The model under review builds one solid part; all positions refer to its coordinate system, in mm. A direction names the side the tool comes from. Round coordinates to 2 decimals unless told otherwise and drop trailing zeros. Loops run counter-clockwise (first coordinate to the right, second up) from the corner with the lowest first, then second, coordinate; pieces in that order, holes last. Notation, with made-up numbers: M 63.5,66 L 76.5,66 A28 cw 76.5,101 Z; hole C -1.75,0 d8. An arc over 180 degrees is marked long. Return JSON: item names as keys, results as strings. Group by question number.
Q1. For faces 1 (the face through (6, 9, 26.5)), 2 (the face through (6, 16, 22.3)), 3 (the face through (6, 0, 8)), list the 3-axis set-ups (+Z, -Z, +X, -X, +Y, -Y) from which the entire face can be reached by the end or side of a thin tool; tool diameter is ignored.
Q2. Consider section C-C (x = 10.75). State the section outline as (y, z) points.
Q3. Consider section A-A (z = 7). State the section outline as (x, y) points, and give its area (3 significant figures).
Q4. Consider section B-B (x = 5.5). Count the separate pieces of the cut face and the enclosed holes in it, and give its area (3 significant figures).
Q5. Clearance check with flat-ended pins moving along their axes: pin 1 Ø6 at (x, y) = (4, -2) entering from +Z; pin 2 Ø2.5 at (x, y) = (3.5, -2) entering from -Z; pin 3 Ø2.5 at (x, y) = (5, 23.5) entering from +Z; pin 4 Ø1.6 at (x, y) = (6, 25) entering from -Z. State where each tip first meets the part, or that it passes through.
Q6. Consider section D-D (z = 23). State the section outline as (x, y) points, and give its area (3 significant figures).
Q7. To check wall thickness, follow line 1 along Y through (x, z) = (5.9, 17.15); line 2 along X through (y, z) = (-2.6, 16.75); line 3 along Z through (x, y) = (1.25, 7). State the ranges of each line that lie inside material, in increasing order.
from build123d import *

# Parameters (mm, degrees)
F0_W     = 11.8
F0_H     = 22.5
F1_DEPTH = 22.3
F4_DEPTH = 2.5
F6_DEPTH = 4.2
F7_R     = 2.45
F8_DEPTH = 3
F9_R     = 0.5


with BuildPart() as f1:
    # F0 (on Top) → F1 (new body)
    with BuildSketch(Plane.XY):
        with Locations((5.9, 11.25)):
            Rectangle(F0_W, F0_H)
    extrude(amount=F1_DEPTH)

    # F3 (on offset) → F4 (join)
    with BuildSketch(Plane.XY.offset(16)):
        Polygon((11.8, 27.4), (0, 27.4), (0, 11.25), (0, -4.9), (11.8, -4.9), align=None)
        with BuildLine():
            ThreePointArc((6.9, -2.6), (5.1928932188, -3.3071067812), (5.9, -1.6))
            ThreePointArc((5.9, -1.6), (6.6071067812, -1.8928932188), (6.9, -2.6))
        make_face(mode=Mode.SUBTRACT)
        with BuildLine():
            ThreePointArc((6.9, 25.1), (6.6071067812, 24.3928932188), (5.9, 24.1))
            ThreePointArc((5.9, 24.1), (5.1928932188, 25.8071067812), (6.9, 25.1))
        make_face(mode=Mode.SUBTRACT)
    extrude(amount=F4_DEPTH)

    # F5 (on face) → F6 (join)
    with BuildSketch(Plane.XY.offset(22.3)):
        with BuildLine():
            ThreePointArc((3.2367553675, 11.1647058824), (2.8099468719, 0.8739108976), (11.8, 5.9))
            ThreePointArc((11.8, 5.9), (10.9260891024, 8.9900531281), (8.5632446325, 11.1647058824))
            ThreePointArc((8.5632446325, 11.1647058824), (5.9, 9.1), (3.2367553675, 11.1647058824))
        make_face()
        with BuildLine():
            ThreePointArc((3.2367553675, 11.1647058824), (5.9, 9.1), (8.5632446325, 11.1647058824))
            ThreePointArc((8.5632446325, 11.1647058824), (5.9, 11.8), (3.2367553675, 11.1647058824))
        make_face()
        with BuildLine():
            ThreePointArc((3.2367553675, 11.1647058824), (5.9, 11.8), (8.5632446325, 11.1647058824))
            ThreePointArc((8.5632446325, 11.1647058824), (8.6282249485, 11.5046181383), (8.65, 11.85))
            ThreePointArc((8.65, 11.85), (5.5546181383, 14.5782249485), (3.2367553675, 11.1647058824))
        make_face()
    extrude(amount=F6_DEPTH)

    # F7 (on face) → F8 (join)
    with BuildSketch(Plane.XY.offset(26.5)):
        with Locations((5.9, 5.9)):
            Circle(F7_R)
    extrude(amount=F8_DEPTH)

    # F9
    f9_edges = [f1.edges().sort_by_distance(p)[0] for p in [
        (11.8, 0, 8),
        (11.8, 0, 20.4),
        (0, 0, 8),
        (0, 0, 20.4),
        (0, 22.5, 20.4),
        (0, 22.5, 8),
        (11.8, 22.5, 8),
        (11.8, 22.5, 20.4),
        (0, -4.9, 17.25),
        (11.8, -4.9, 17.25),
        (11.8, 27.4, 17.25),
        (0, 27.4, 17.25),
    ]]
    fillet(f9_edges, radius=F9_R)


solid = f1.part
Values:
{
 "1": {"face 1": "+Z", "face 2": "+Z, +Y", "face 3": "-Z, +X, -X, -Y"},
 "2": {"outline": "M -4.9,16 L 0,16 L 0,0 L 22.5,0 L 22.5,16 L 27.4,16 L 27.4,18.5 L 22.5,18.5 L 22.5,22.3 L 9.26,22.3 L 9.26,26.5 L 2.54,26.5 L 2.54,22.3 L 0,22.3 L 0,18.5 L -4.9,18.5 Z"},
 "3": {"outline": "M 0,0.5 A0.5 ccw 0.5,0 L 11.3,0 A0.5 ccw 11.8,0.5 L 11.8,22 A0.5 ccw 11.3,22.5 L 0.5,22.5 A0.5 ccw 0,22 Z", "area": "265 mm2"},
 "4": {"separate pieces": "3", "enclosed holes": "0", "area": "593 mm2"},
 "5": {"pin 1": "stops at z = 26.5", "pin 2": "stops at z = 16", "pin 3": "stops at z = 22.3", "pin 4": "passes through"},
 "6": {"outline": "M 3.24,11.16 A5.9 ccw long 8.56,11.16 A2.75 ccw long Z", "area": "123 mm2"},
 "7": {"line 1": "y = -4.9 to -3.6, -1.6 to 24.1, 26.1 to 27.4", "line 2": "x = 0 to 4.9, 6.9 to 11.8", "line 3": "z = 0 to 26.5"}
}
